from build123d import *

# Parameters (mm, degrees)
SKETCH1_W               = 2.7
SKETCH1_H               = 2
CUT_EXTRUDE1_DEPTH      = 25
CUT_EXTRUDE1_DEPTH_BACK = 25
SKETCH2_R               = 2.15
CUT_EXTRUDE3_DEPTH      = 25
CUT_EXTRUDE3_DEPTH_BACK = 3
SKETCH2_4_R             = 4.25
BOSS_EXTRUDE1_DEPTH     = 1
SKETCH4_W               = 7.5
SKETCH4_H               = 7.5
BOSS_EXTRUDE2_DEPTH     = 13
FILLET1_START           = 9
FILLET1_DEPTH           = 5
FILLET2_R               = 1
CUT_EXTRUDE4_REACH      = 39.082
SKETCH5_R               = 2.15


with BuildPart() as part:
    # Sketch1 → Revolve1 (revolve)
    with BuildSketch(Plane(origin=(0, 0, 0), x_dir=(1, 0, 0), z_dir=(0, 1, 0)), mode=Mode.PRIVATE) as revolve1_sk:
        Polygon((16, 0), (2.7, 0), (2.7, -12), (2.7, -14), (12.4, -14), (12.4, -8), (16, -8), align=None)
        with Locations((1.35, -13)):
            Rectangle(SKETCH1_W, SKETCH1_H)
    revolve(revolve1_sk.sketch.rotate(Axis((0, 0, 0), (0, 0, 1)), 180), axis=Axis((0, 0, 0), (0, 0, 1)))

    # Sketch2 → Cut-Extrude1 (cut, two sides: drawn at the far end of the back side and taken through both)
    with BuildSketch(Plane.XY.offset(8).offset(-CUT_EXTRUDE1_DEPTH_BACK)):
        with Locations((-8, 8)):
            Circle(SKETCH2_R)
        with Locations((8, 8)):
            Circle(SKETCH2_R)
        with Locations((8, -8)):
            Circle(SKETCH2_R)
        with Locations((-8, -8)):
            Circle(SKETCH2_R)
    extrude(amount=CUT_EXTRUDE1_DEPTH + CUT_EXTRUDE1_DEPTH_BACK, mode=Mode.SUBTRACT)

    # Sketch2<4> → Cut-Extrude3 (cut, two sides: drawn at the far end of the back side and taken through both)
    with BuildSketch(Plane.XY.offset(8).offset(-CUT_EXTRUDE3_DEPTH_BACK)):
        with Locations((-8, 8)):
            Circle(SKETCH2_4_R)
        with Locations((8, 8)):
            Circle(SKETCH2_4_R)
        with Locations((8, -8)):
            Circle(SKETCH2_4_R)
        with Locations((-8, -8)):
            Circle(SKETCH2_4_R)
    extrude(amount=CUT_EXTRUDE3_DEPTH + CUT_EXTRUDE3_DEPTH_BACK, mode=Mode.SUBTRACT)

    # Sketch3 → Boss-Extrude1 (add)
    with BuildSketch(Plane.XY.offset(8)):
        with BuildLine():
            ThreePointArc((5.244985625, 11.236108125), (5.769768323, 11.617812415), (6.346544904, 11.915173846))
            ThreePointArc((6.346544904, 11.915173846), (0, 13.5), (-6.346544904, 11.915173846))
            ThreePointArc((-6.346544904, 11.915173846), (-5.769768323, 11.617812415), (-5.244985625, 11.236108125))
            ThreePointArc((-5.244985625, 11.236108125), (0, 12.4), (5.244985625, 11.236108125))
        make_face()
        with BuildLine():
            ThreePointArc((-11.236108125, 5.244985625), (-11.617812415, 5.769768323), (-11.915173846, 6.346544904))
            ThreePointArc((-11.915173846, 6.346544904), (-13.5, 0), (-11.915173846, -6.346544904))
            ThreePointArc((-11.915173846, -6.346544904), (-11.617812415, -5.769768323), (-11.236108125, -5.244985625))
            ThreePointArc((-11.236108125, -5.244985625), (-12.4, 0), (-11.236108125, 5.244985625))
        make_face()
        with BuildLine():
            ThreePointArc((-6.346544904, -11.915173846), (0, -13.5), (6.346544904, -11.915173846))
            ThreePointArc((6.346544904, -11.915173846), (5.769768323, -11.617812415), (5.244985625, -11.236108125))
            ThreePointArc((5.244985625, -11.236108125), (0, -12.4), (-5.244985625, -11.236108125))
            ThreePointArc((-5.244985625, -11.236108125), (-5.769768323, -11.617812415), (-6.346544904, -11.915173846))
        make_face()
        with BuildLine():
            ThreePointArc((11.915173846, -6.346544904), (13.097802238, -3.270714989), (13.5, 0))
            ThreePointArc((13.5, 0), (13.097802238, 3.270714989), (11.915173846, 6.346544904))
            ThreePointArc((11.915173846, 6.346544904), (11.617812415, 5.769768323), (11.236108125, 5.244985625))
            ThreePointArc((11.236108125, 5.244985625), (12.4, 0), (11.236108125, -5.244985625))
            ThreePointArc((11.236108125, -5.244985625), (11.617812415, -5.769768323), (11.915173846, -6.346544904))
        make_face()
    extrude(amount=BOSS_EXTRUDE1_DEPTH)

    # Sketch4 → Boss-Extrude2 (add)
    with BuildSketch(Plane.XY.offset(14)):
        with BuildLine():
            Line((-3.75, 11.819369696), (-3.75, 3.75))
            Line((-3.75, 3.75), (3.75, 3.75))
            Line((3.75, 3.75), (3.75, 11.819369696))
            ThreePointArc((3.75, 11.819369696), (0, 12.4), (-3.75, 11.819369696))
        make_face()
        Rectangle(SKETCH4_W, SKETCH4_H)
        with BuildLine():
            Line((-3.75, 3.75), (-11.819369696, 3.75))
            ThreePointArc((-11.819369696, 3.75), (-12.4, 0), (-11.819369696, -3.75))
            Line((-11.819369696, -3.75), (-3.75, -3.75))
            Line((-3.75, -3.75), (-3.75, 3.75))
        make_face()
        with BuildLine():
            Line((3.75, -3.75), (-3.75, -3.75))
            Line((-3.75, -3.75), (-3.75, -11.819369696))
            ThreePointArc((-3.75, -11.819369696), (0, -12.4), (3.75, -11.819369696))
            Line((3.75, -11.819369696), (3.75, -3.75))
        make_face()
        with BuildLine():
            Line((11.819369696, 3.75), (3.75, 3.75))
            Line((3.75, 3.75), (3.75, -3.75))
            Line((3.75, -3.75), (11.819369696, -3.75))
            ThreePointArc((11.819369696, -3.75), (12.253982704, -1.897342322), (12.4, 0))
            ThreePointArc((12.4, 0), (12.253982704, 1.897342322), (11.819369696, 3.75))
        make_face()
    extrude(amount=BOSS_EXTRUDE2_DEPTH)

    # Fillet1: read off the stored shape, not the designer's step
    # Fillet1 outline → Fillet1 (cut)
    with BuildSketch(Plane.XY.offset(FILLET1_START)):
        with BuildLine():
            ThreePointArc((-10.286897346, -4.417738071), (-11.160201718, -4.516996035), (-11.774551439, -3.8884365))
            ThreePointArc((-11.774551439, -3.8884365), (-11.525305626, -4.574639902), (-11.236108125, -5.244985625))
            ThreePointArc((-11.236108125, -5.244985625), (-10.792307645, -4.796015291), (-10.286897346, -4.417738071))
        make_face()
        with BuildLine():
            ThreePointArc((-11.236108125, 5.244985625), (-11.525305626, 4.574639902), (-11.774551439, 3.8884365))
            ThreePointArc((-11.774551439, 3.8884365), (-11.160201718, 4.516996035), (-10.286897346, 4.417738071))
            ThreePointArc((-10.286897346, 4.417738071), (-10.792307645, 4.796015291), (-11.236108125, 5.244985625))
        make_face()
        with BuildLine():
            ThreePointArc((-4.417738071, -10.286897346), (-4.796015291, -10.792307645), (-5.244985625, -11.236108125))
            ThreePointArc((-5.244985625, -11.236108125), (-4.574639902, -11.525305626), (-3.8884365, -11.774551439))
            ThreePointArc((-3.8884365, -11.774551439), (-4.516996035, -11.160201718), (-4.417738071, -10.286897346))
        make_face()
        with BuildLine():
            ThreePointArc((-3.8884365, 11.774551439), (-4.574639902, 11.525305626), (-5.244985625, 11.236108125))
            ThreePointArc((-5.244985625, 11.236108125), (-4.796015291, 10.792307645), (-4.417738071, 10.286897346))
            ThreePointArc((-4.417738071, 10.286897346), (-4.516996035, 11.160201718), (-3.8884365, 11.774551439))
        make_face()
        with BuildLine():
            ThreePointArc((4.417738071, -10.286897346), (4.516996035, -11.160201718), (3.8884365, -11.774551439))
            ThreePointArc((3.8884365, -11.774551439), (4.574639902, -11.525305626), (5.244985625, -11.236108125))
            ThreePointArc((5.244985625, -11.236108125), (4.796015291, -10.792307645), (4.417738071, -10.286897346))
        make_face()
        with BuildLine():
            ThreePointArc((5.244985625, 11.236108125), (4.574639902, 11.525305626), (3.8884365, 11.774551439))
            ThreePointArc((3.8884365, 11.774551439), (4.516996035, 11.160201718), (4.417738071, 10.286897346))
            ThreePointArc((4.417738071, 10.286897346), (4.796015291, 10.792307645), (5.244985625, 11.236108125))
        make_face()
        with BuildLine():
            ThreePointArc((11.774551439, -3.8884365), (11.160201718, -4.516996035), (10.286897346, -4.417738071))
            ThreePointArc((10.286897346, -4.417738071), (10.792307645, -4.796015291), (11.236108125, -5.244985625))
            ThreePointArc((11.236108125, -5.244985625), (11.525305626, -4.574639902), (11.774551439, -3.8884365))
        make_face()
        with BuildLine():
            ThreePointArc((11.236108125, 5.244985625), (10.792307645, 4.796015291), (10.286897346, 4.417738071))
            ThreePointArc((10.286897346, 4.417738071), (11.160201718, 4.516996035), (11.774551439, 3.8884365))
            ThreePointArc((11.774551439, 3.8884365), (11.525305626, 4.574639902), (11.236108125, 5.244985625))
        make_face()
    extrude(amount=FILLET1_DEPTH, mode=Mode.SUBTRACT)

    # Fillet2
    # the kernel refuses this fillet: 1 mm, written as the material it takes off along each edge
    with BuildSketch(Plane(origin=(6.346544904, 11.915173846, 8), x_dir=(-0.9128071588111344, 0.4083908554597477, 0), z_dir=(0, 0, 1)), Plane(origin=(-11.915173846, 6.346544904, 8), x_dir=(-0.4083908554599063, -0.9128071588110634, 0), z_dir=(0, 0, 1)), Plane(origin=(-6.346544904, -11.915173846, 8), x_dir=(0.9128071588110586, -0.408390855459917, 0), z_dir=(0, 0, 1)), Plane(origin=(11.915173846, -6.346544904, 8), x_dir=(0.4083908554598645, 0.9128071588110821, 0), z_dir=(0, 0, 1))) as fillet2_piece_1:
        with BuildLine():
            CenterArc((1.785571343, 0.997639029), FILLET2_R, 158.772199303, 115.165734994)
            ThreePointArc((0.853423117, 1.359715932), (0.491495222, 0.639196623), (0, 0))
            ThreePointArc((0, 0), (0.927123582, -0.031873112), (1.854247164, 0))
        make_face()
    extrude(amount=5.63561791, mode=Mode.SUBTRACT)
    with BuildSketch(Plane(origin=(-6.346544904, 11.915173846, 8), x_dir=(0.9128071588110631, 0.4083908554599068, 0), z_dir=(0, 0, 1)), Plane(origin=(-11.915173846, -6.346544904, 8), x_dir=(-0.4083908554599002, 0.912807158811066, 0), z_dir=(0, 0, 1)), Plane(origin=(6.346544904, -11.915173846, 8), x_dir=(-0.9128071588111399, -0.40839085545973536, 0), z_dir=(0, 0, 1)), Plane(origin=(11.915173846, 6.346544904, 8), x_dir=(0.40839085545986265, -0.912807158811083, 0), z_dir=(0, 0, 1))) as fillet2_piece_2:
        with BuildLine():
            CenterArc((1.785571343, -0.997639029), FILLET2_R, 86.062065704, 115.165734994)
            ThreePointArc((0.853423117, -1.359715932), (0.491495222, -0.639196623), (0, 0))
            ThreePointArc((0, 0), (0.927123582, 0.031873112), (1.854247164, 0))
        make_face()
    extrude(amount=5.63561791, mode=Mode.SUBTRACT)

    # Sketch5 → Cut-Extrude4 (cut, up to next)
    with BuildSketch(Plane(origin=(0, 3.75, 0), x_dir=(1, 0, 0), z_dir=(0, 1, 0)), mode=Mode.PRIVATE) as cut_extrude4_sk1:
        with Locations(Location((-8, -22, 0), (0, 0, 270))):
            Circle(SKETCH5_R)
    cut_extrude4_tool1 = extrude(cut_extrude4_sk1.sketch, amount=-CUT_EXTRUDE4_REACH, mode=Mode.PRIVATE) & part.part
    # Sketch5 → Cut-Extrude4 (cut, up to next)
    with BuildSketch(Plane(origin=(0, 3.75, 0), x_dir=(1, 0, 0), z_dir=(0, 1, 0)), mode=Mode.PRIVATE) as cut_extrude4_sk2:
        with Locations(Location((8, -22, 0), (0, 0, 270))):
            Circle(SKETCH5_R)
    cut_extrude4_tool2 = extrude(cut_extrude4_sk2.sketch, amount=-CUT_EXTRUDE4_REACH, mode=Mode.PRIVATE) & part.part
    add(cut_extrude4_tool1.solids().sort_by_distance((-8, 3.75, 22))[0], mode=Mode.SUBTRACT)
    add(cut_extrude4_tool2.solids().sort_by_distance((8, 3.75, 22))[0], mode=Mode.SUBTRACT)


solid = part.part
For this review, take the finished solid that the model builds, in its own axes (mm). A direction names the side the tool comes from. Coordinates: 2 decimals unless noted, no trailing zeros. Order: outer loops, then holes, each group sorted by start corner. A loop starts at its lowest first (then second) coordinate and runs counter-clockwise, first axis right, second up. Notation, with made-up numbers: (34, 48.25) - (60, 48.25) arc R27 cw to (60, 85.25) - close; hole circle Ø6 at (-35.75, -17.75). An arc over 180 degrees is marked (long way). Use one line per item in the form item = value.
Q1. Consider section D-D (y = 8.5). Give the number of separate pieces and of enclosed holes in the cut face, then the cut area to 3 significant figures.
Checked values:
separate_pieces = 3
enclosed_holes = 0
area = 267 mm2
Q2. For P1, Ø1.5, axis at y = -8, z = 14.5, coming from the -X side; P2, Ø1.5, axis at x = 12.5, y = 2.5, coming from the -Z side; P3, Ø10, axis at x = -10, z = 8, coming from the -Y side; P4, Ø2.5, axis at y = 8, z = 22.5, coming from the +X side, all flat-tipped, find the tip position at first contact; note any pin that passes through.
Checked values:
P1 = -3.79
P2 = 0
P3 = -15.2
P4 = 3.75
Q3. Consider section B-B (x = -9). Give the boundary of the cut face in (y, z).
Checked values:
outline = (-13.23, 0) - (-9.9, 0) - (-9.9, 5) - (-12.13, 5) - (-12.13, 8) - (-13.23, 8) - close; (-6.1, 0) - (6.1, 0) - (6.1, 5) - (3.87, 5) - (3.87, 14) - (3.75, 14) - (3.75, 20.1) - (-3.75, 20.1) - (-3.75, 14) - (-3.87, 14) - (-3.87, 5) - (-6.1, 5) - close; (-3.75, 23.9) - (3.75, 23.9) - (3.75, 27) - (-3.75, 27) - close; (9.9, 0) - (13.23, 0) - (13.23, 8) - (12.13, 8) - (12.13, 5) - (9.9, 5) - close
Q4. Consider section C-C (x = 0). Give the boundary of the cut face in (y, z).
Checked values:
outline = (-16, 0) - (-2.7, 0) - (-2.7, 12) - (2.7, 12) - (2.7, 0) - (16, 0) - (16, 8) - (13.5, 8) - (13.5, 9) - (12.4, 9) - (12.4, 27) - (-12.4, 27) - (-12.4, 9) - (-13.5, 9) - (-13.5, 8) - (-16, 8) - close
Q5. For faces 1 (the cylindrical face through (-4.52, 11.15, 11.46)), 2 (the flat face through (-4, 11, 14)), 3 (the cylindrical face through (-11.15, -4.52, 11.46)), 4 (the flat face through (4, -10, 14)), list the 3-axis set-ups (+Z, -Z, +X, -X, +Y, -Y) from which the entire face can be reached by the end or side of a thin tool; tool diameter is ignored.
Checked values:
face_1 = +Z, -X
face_2 = +Z, -X, +Y
face_3 = +Z, -Y
face_4 = +Z, +X, -Y
Q6. Consider section A-A (z = 22). Give the boundary of the cut face in (x, y), then the cut area to 3 significant figures.
Checked values:
outline = (-11.82, -3.75) - (-10.15, -3.75) - (-10.15, 3.75) - (-11.82, 3.75) arc R12.4 ccw to start; (-5.85, -3.75) - (-3.75, -3.75) - (-3.75, -11.82) arc R12.4 ccw to (3.75, -11.82) - (3.75, -3.75) - (5.85, -3.75) - (5.85, 3.75) - (3.75, 3.75) - (3.75, 11.82) arc R12.4 ccw to (-3.75, 11.82) - (-3.75, 3.75) - (-5.85, 3.75) - close; (10.15, -3.75) - (11.82, -3.75) arc R12.4 ccw to (11.82, 3.75) - (10.15, 3.75) - close
area = 245 mm2
Q7. Draft analysis for pull direction X (two halves, no side actions). For faces 5 (the flat face through (10, -10, 5)), 6 (the flat face through (-3.75, -8, 20)), 7 (the flat face through (-10, 4, 14)), state which applies: +X half, -X half, draft (parallel to the pull), parting line (faces both ways), or undercut.
Checked values:
face_5 = undercut
face_6 = -X half
face_7 = draft
Q8. For probe 1 along Y at (x, z) = (8.5, 4.5); probe 2 along Y at (x, z) = (-8, 1.95); probe 3 along X at (y, z) = (1.5, 21), list the stretches that pass through material, from the lowest coordinate up. Write a range as from..to.
Checked values:
probe_1 = -13.56..-10.09, -5.91..5.91, 10.09..13.56
probe_2 = -13.86..-10.15, -5.85..5.85, 10.15..13.86
probe_3 = -12.31..-9.9, -6.1..6.1, 9.9..12.31
